Verification items for the finished model (mm, model axes). Coordinates: 2 decimals unless noted, no trailing zeros. Write each loop counter-clockwise with the first axis right and the second up, starting at its lowest first coordinate (ties: lowest second). Pieces come first, ordered by that corner, then holes. Notation, with made-up numbers: (74, 81) -> (79, 81) arc R29 cw to (79, 112) -> close; hole circle Ø3 at (26.5, 38). An arc over 180 degrees is marked (long way). Answer in a Markdown table with one row per item.
```python
from build123d import *

# Parameters (mm, degrees)
ESQUISSE1_W             = 56.4
ESQUISSE1_H             = 56.4
ESQUISSE1_R             = 2
BOSS_EXTRU_1_DEPTH      = 10
ESQUISSE2_R             = 19.05
ENL_V_MAT_EXTRU_1_DEPTH = 10
CONG_1_R                = 2


with BuildPart() as part:
    # Esquisse1 → Boss.-Extru.1 (new body)
    with BuildSketch(Plane.XY):
        Rectangle(ESQUISSE1_W, ESQUISSE1_H)
        with Locations((23.57, 23.57)):
            Circle(ESQUISSE1_R, mode=Mode.SUBTRACT)
        with Locations(Location((-23.57, 23.57, 0), (0, 0, 180))):
            Circle(ESQUISSE1_R, mode=Mode.SUBTRACT)
        with Locations(Location((23.57, -23.57, 0), (0, 0, 180))):
            Circle(ESQUISSE1_R, mode=Mode.SUBTRACT)
        with Locations((-23.57, -23.57)):
            Circle(ESQUISSE1_R, mode=Mode.SUBTRACT)
    extrude(amount=BOSS_EXTRU_1_DEPTH)

    # Esquisse2 → Enlèv. mat.-Extru.1 (cut)
    with BuildSketch(Plane.XY.offset(10)):
        Circle(ESQUISSE2_R)
    extrude(amount=-ENL_V_MAT_EXTRU_1_DEPTH, mode=Mode.SUBTRACT)

    # Congé1
    cong_1_edges = [part.edges().sort_by_distance(p)[0] for p in [
        (28.2, -28.2, 5),
        (-28.2, -28.2, 5),
        (-28.2, 28.2, 5),
        (28.2, 28.2, 5),
    ]]
    fillet(cong_1_edges, radius=CONG_1_R)


solid = part.part
```
1. Sectioned sample at A-A, the plane z = 8.5. Record the cut outline in (x, y), and give its area (3 significant figures).
Findings below:
| item | result |
|---|---|
| outline | (-28.2, -26.2) arc R2 ccw to (-26.2, -28.2) -> (26.2, -28.2) arc R2 ccw to (28.2, -26.2) -> (28.2, 26.2) arc R2 ccw to (26.2, 28.2) -> (-26.2, 28.2) arc R2 ccw to (-28.2, 26.2) -> close; hole circle Ø4 at (-23.57, -23.57); hole circle Ø4 at (-23.57, 23.57); hole circle Ø38.1 at (0, 0); hole circle Ø4 at (23.57, -23.57); hole circle Ø4 at (23.57, 23.57) |
| area | 1,990 mm² |
2. Sectioned sample at B-B, the plane x = -23.57. Record the cut outline in (y, z), and give its area (3 significant figures).
Findings below:
| item | result |
|---|---|
| outline | (-28.2, 0) -> (-25.57, 0) -> (-25.57, 10) -> (-28.2, 10) -> close; (-21.57, 0) -> (21.57, 0) -> (21.57, 10) -> (-21.57, 10) -> close; (25.57, 0) -> (28.2, 0) -> (28.2, 10) -> (25.57, 10) -> close |
| area | 484 mm² |
3. Go/stop test with a flat-tipped pin: pin 1 (2.5 mm diameter, centred on x = -23.57, y = 23.57, fed in from -Z). Record where the tip stops, or that it passes through.
Findings below:
| item | result |
|---|---|
| pin 1 | passes through |
4. Sectioned sample at D-D, the plane y = 0. Record the cut outline in (x, z), and give its area (3 significant figures).
Findings below:
| item | result |
|---|---|
| outline | (-28.2, 0) -> (-19.05, 0) -> (-19.05, 10) -> (-28.2, 10) -> close; (19.05, 0) -> (28.2, 0) -> (28.2, 10) -> (19.05, 10) -> close |
| area | 183 mm² |
5. Release check for a two-part mould opening along X. For faces 1 (the face through (28.2, 0, 5)), 2 (the face through (21.572, 23.658, 4.93)), 3 (the face through (-27.63, -27.6, 5.07)), 4 (the face through (25.568, -23.658, 4.93)) record: released by +X, released by -X, zero draft, split by the parting line, or undercut.
Findings below:
| item | result |
|---|---|
| face 1 | released by +X |
| face 2 | undercut |
| face 3 | released by -X |
| face 4 | undercut |
6. Material ranges on probe 1 along Y at (x, z) = (-23.57, 7); probe 2 along Y at (x, z) = (25, 8), recorded low to high. Write a range as from..to.
Findings below:
| item | result |
|---|---|
| probe 1 | y = -28.2..-25.57, -21.57..21.57, 25.57..28.2 |
| probe 2 | y = -28.2..-24.97, -22.17..22.17, 24.97..28.2 |
